Design review of the part built by this model. Coordinates are the model's own, in mm. A direction names the side the tool comes from. Give positions to 0.01 mm unless a question says otherwise; leave off trailing zeros. Loops run counter-clockwise (first coordinate to the right, second up) from the corner with the lowest first, then second, coordinate; pieces in that order, holes last. Notation, with made-up numbers: M 9.5,47 L 30.5,47 A12 ccw 30.5,65 Z; hole C 44,33 d6. An arc over 180 degrees is marked long. Use a Markdown table: item, result. Add a question column.
(1) Draft analysis for pull direction X (two halves, no side actions). For faces 6 (the face through (-0.15, 0.52, 3.07)), 7 (the face through (0.1, 0.5, 6.35)), 8 (the face through (-0.99, 2, -2)), 9 (the face through (3.81, 0.5, -0.1)), state which applies: pulls with the +X half, pulls with the -X half, needs draft (parallel to the pull), parting line crosses it, or undercut.
(2) Add section A-A, the plane x = -0.01. Give the boundary of the cut face in (y, z).
(3) Add section D-D, the plane x = 2.5. Give the boundary of the cut face in (y, z), then the cut area to 3 significant figures.
(4) Add section C-C, the plane y = 0.6. Give the boundary of the cut face in (x, z).
(5) For probe 1 along Z at (x, y) = (-0.01, 0.6); probe 2 along X at (y, z) = (0.7, 4.15); probe 3 along Y at (x, z) = (-2.75, 0.5), list the stretches that pass through material, from the lowest coordinate up.
(6) Add section B-B, the plane z = 4.15. Give the boundary of the cut face in (x, y), then the cut area to 3 significant figures.
(7) Insertion check: pin 1 Ø2.5 at (x, z) = (-1.5, 3) entering from +Y; pin 2 Ø0.8 at (x, y) = (-0.5, 2) entering from -Z; pin 3 Ø1.3 at (x, z) = (-0.01, 4.15) entering from +Y; pin 4 Ø0.8 at (y, z) = (2, -2) entering from +X. Each pin has a flat end and moves straight along its axis. Give the tip position at first contact, or say it passes through.
(8) For faces 1 (the face through (0, 2.52, -2)), 2 (the face through (0, 2, -3.8)), 3 (the face through (0, 2, -0.8)), 4 (the face through (0, 0, 0)), 5 (the face through (1.01, 2, -2)), list the 3-axis set-ups (+Z, -Z, +X, -X, +Y, -Y) from which the entire face can be reached by the end or side of a thin tool; tool diameter is ignored.
Autodesk Inventor part; units mm, degrees
ref_plane "YZ Plane" through (0, 0, 0) normal (1, 0, 0) x (0, 1, 0)
ref_plane "XZ Plane" through (0, 0, 0) normal (0, 1, 0) x (-1, 0, 0)
ref_plane "XY Plane" through (0, 0, 0) normal (0, 0, 1) x (1, 0, 0)
sketch "Sketch1" plane through (0, 0, 0) normal (0, 1, 0) x (-1, 0, 0)
  line L0 (-3.81, 6.35) -> (3.81, 6.35)
  line L1 (3.81, 6.35) -> (3.81, -6.35)
  line L2 (3.81, -6.35) -> (-3.81, -6.35)
  line L3 (-3.81, -6.35) -> (-3.81, 6.35)
  line L4 (-3.81, 6.35) -> (3.81, -6.35) construction
  line L5 (3.81, 6.35) -> (-3.81, -6.35) construction
  point P0 (0, 0)
  dimension "d0" = 12.7
  dimension "d1" = 7.62
extrude "Extrusion1" add sketch "Sketch1" along normal blind 2.52
sketch "Sketch2" plane through (0, 2.52, 0) normal (0, 1, 0) x (1, 0, 0)
  circle A0 centre (-0.01, -4.15) radius 1.09
  line L0 (-3.81, -6.35) -> (3.81, -6.35)
  line L1 (0.99, 3.35) -> (-1.01, 3.35)
  line L2 (-1.01, 3.35) -> (-1.01, 0.35)
  line L3 (-1.01, 0.35) -> (0.99, 0.35)
  line L4 (0.99, 0.35) -> (0.99, 3.35)
  line L5 (0.99, 3.35) -> (-1.01, 0.35) construction
  line L6 (-1.01, 3.35) -> (0.99, 0.35) construction
  line L7 (-3.81, 6.35) -> (-3.81, -6.35)
  line L8 (3.81, 6.35) -> (-3.81, 6.35)
  point P0 (0, 0)
  point P1 (0, -6.35)
  point P2 (-0.01, 1.85)
  dimension "d4" = 2.18
  dimension "d5" = 2.2
  dimension "d6" = 3
  dimension "d7" = 2
  dimension "d16" = 3.8
  dimension "d17" = 4.5
  dimension "d18" = 3.8
extrude "Extrusion2" cut sketch "Sketch2" against normal through all contours A0
sketch "Sketch3" plane through (0, 2.52, 0) normal (0, 1, 0) x (1, 0, 0)
  line L0 (1.01, 0.8) -> (-0.99, 0.8)
  line L1 (-0.99, 0.8) -> (-0.99, 3.8)
  line L2 (-0.99, 3.8) -> (1.01, 3.8)
  line L3 (1.01, 3.8) -> (1.01, 0.8)
  line L4 (1.01, 0.8) -> (-0.99, 3.8) construction
  line L5 (-0.99, 0.8) -> (1.01, 3.8) construction
  line L6 (3.81, -6.35) -> (3.81, 6.35)
  line L7 (-3.81, -6.35) -> (3.81, -6.35)
  line L8 (3.81, 6.35) -> (-3.81, 6.35)
  line L9 (-3.81, -6.35) -> (3.81, -6.35)
  line L10 (3.81, -6.35) -> (3.81, 6.35)
  line L11 (3.81, 6.35) -> (-3.81, 6.35)
  line L12 (-3.81, 6.35) -> (-3.81, -6.35)
  point P0 (0, 0)
  point P1 (0.01, 2.3)
  dimension "d10" = 3
  dimension "d11" = 2
  dimension "d12" = 2.3
  dimension "d13" = 3.8
extrude "Extrusion3" cut sketch "Sketch3" against normal blind 1.5
properties part number "lightSensor"
Established:
| question | item | result |
|---|---|---|
| 1 | face 6 | undercut |
| 1 | face 7 | needs draft |
| 1 | face 8 | pulls with the -X half |
| 1 | face 9 | pulls with the +X half |
| 2 | outline | M 0,-6.35 L 1.02,-6.35 L 1.02,-3.8 L 2.52,-3.8 L 2.52,-0.8 L 1.02,-0.8 L 1.02,3.06 L 0,3.06 Z; M 0,5.24 L 1.02,5.24 L 1.02,6.35 L 0,6.35 Z |
| 3 | outline | M 0,-6.35 L 1.02,-6.35 L 1.02,6.35 L 0,6.35 Z |
| 3 | area | 13.0 mm^2 |
| 4 | outline | M -3.81,-6.35 L 3.81,-6.35 L 3.81,6.35 L -3.81,6.35 Z; hole C -0.01,4.15 d2.18 |
| 5 | probe 1 | -6.35 to 3.06, 5.24 to 6.35 |
| 5 | probe 2 | -3.81 to -1.1, 1.08 to 3.81 |
| 5 | probe 3 | 0 to 1.02 |
| 6 | outline | M -3.81,0 L -1.1,0 L -1.1,1.02 L -3.81,1.02 Z; M 1.08,0 L 3.81,0 L 3.81,1.02 L 1.08,1.02 Z |
| 6 | area | 5.55 mm^2 |
| 7 | pin 1 | y = 1.02 |
| 7 | pin 2 | z = -3.8 |
| 7 | pin 3 | through |
| 7 | pin 4 | x = 1.01 |
| 8 | face 1 | +Z, -Z, +X, -X, +Y |
| 8 | face 2 | -Z, +X, -X, +Y |
| 8 | face 3 | +Z, +X, -X, +Y |
| 8 | face 4 | +Z, -Z, +X, -X, -Y |
| 8 | face 5 | +Z, -Z, +X, +Y |
